```python
from build123d import *

# Parameters (mm, degrees)
ESQUISSE1_W                  = 220
ESQUISSE1_H                  = 200
BOSS_EXTRU_1_DEPTH           = 3
ESQUISSE2_R                  = 17.5
ENL_V_MAT_EXTRU_1_DEPTH      = 149.690954668
R_P_TITION_CIRCULAIRE1_COUNT = 6
R_P_TITION_CIRCULAIRE1_ANGLE = 120
EMPREINTE1_START             = 82
EMPREINTE1_OUTLINE_W         = 40
EMPREINTE1_OUTLINE_H         = 3
EMPREINTE1_DEPTH             = 3
EMPREINTE1_START_2           = 38.6
EMPREINTE1_2_OUTLINE_W       = 3
EMPREINTE1_2_OUTLINE_H       = 3
EMPREINTE1_2_DEPTH           = 33


# Read off the part's stored shape, not the designer's step: Empreinte1
with BuildPart() as part:
    # Esquisse1 → Boss.-Extru.1 (new body)
    with BuildSketch(Plane.XY):
        Rectangle(ESQUISSE1_W, ESQUISSE1_H)
    extrude(amount=BOSS_EXTRU_1_DEPTH)

    # Esquisse2 → Enlèv. mat.-Extru.1 (cut, through all)
    with BuildSketch(Plane.XY.offset(3)):
        with Locations((-86.602540378, -15)):
            Circle(ESQUISSE2_R)
    enl_v_mat_extru_1 = extrude(amount=-ENL_V_MAT_EXTRU_1_DEPTH, mode=Mode.SUBTRACT)

    # Répétition circulaire1: Enlèv. mat.-Extru.1 ×6 about axis
    r_p_tition_circulaire1_axis = Axis((0, 35, 0), (0, 0, 1))
    for i in range(1, R_P_TITION_CIRCULAIRE1_COUNT):
        add(enl_v_mat_extru_1.rotate(r_p_tition_circulaire1_axis, i * R_P_TITION_CIRCULAIRE1_ANGLE / (R_P_TITION_CIRCULAIRE1_COUNT - 1)), mode=Mode.SUBTRACT)

    # Empreinte1 outline → Empreinte1 (cut)
    with BuildSketch(Plane(origin=(0, 0, 0), x_dir=(1, 0, 0), z_dir=(0, 1, 0)).offset(EMPREINTE1_START)):
        with Locations((-53.7, -1.5)):
            Rectangle(EMPREINTE1_OUTLINE_W, EMPREINTE1_OUTLINE_H)
        with Locations((7.3, -1.5)):
            Rectangle(EMPREINTE1_OUTLINE_W, EMPREINTE1_OUTLINE_H)
    extrude(amount=EMPREINTE1_DEPTH, mode=Mode.SUBTRACT)

    # Empreinte1 2 outline → Empreinte1 2 (cut)
    with BuildSketch(Plane(origin=(0, 0, 0), x_dir=(1, 0, 0), z_dir=(0, 1, 0)).offset(EMPREINTE1_START_2)):
        with Locations((-92.2, -1.5)):
            Rectangle(EMPREINTE1_2_OUTLINE_W, EMPREINTE1_2_OUTLINE_H)
        with Locations((45.8, -1.5)):
            Rectangle(EMPREINTE1_2_OUTLINE_W, EMPREINTE1_2_OUTLINE_H)
    extrude(amount=EMPREINTE1_2_DEPTH, mode=Mode.SUBTRACT)


solid = part.part
```
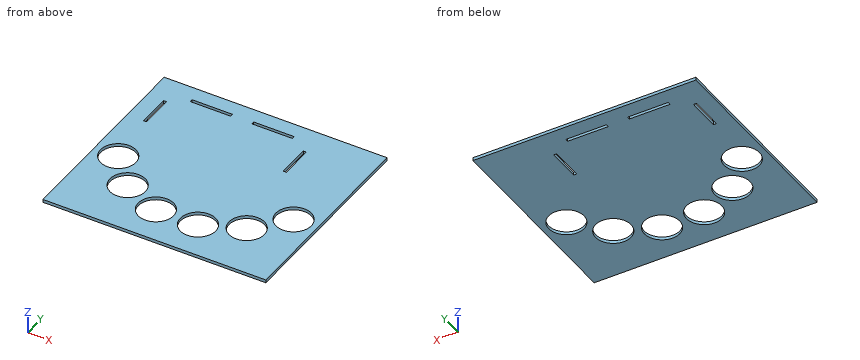
Geometry check sheet. Reference: the model listing, model coordinates, mm. Round coordinates to 2 decimals unless told otherwise and drop trailing zeros. Loops run counter-clockwise (first coordinate to the right, second up) from the corner with the lowest first, then second, coordinate; pieces in that order, holes last. Notation, with made-up numbers: M -19.5,-37.75 L 7.5,-37.75 A13 cw 7.5,-20.75 Z; hole C 71.5,52 d11. An arc over 180 degrees is marked long. Return JSON: item names as keys, results as strings. Group by question number.
(1) Section check B-B, the plane z = 1.25. Give the number of separate pieces and of enclosed holes in the cut face, and give its area (3 significant figures).
(2) Scan lines: line 1 along X through (y, z) = (47, 2.6); line 2 along Y through (x, z) = (10, 0.25); line 3 along Y through (x, z) = (-1.5, 2.8). Record each from-to range of solid material in increasing order. Write a range as [from, to].
(3) Section check A-A, the plane y = 56. Enter the section's corners in (x, z).
(4) Section check C-C, the plane x = 22. Enter the section's corners in (y, z), and give its area (3 significant figures).
(5) Section check D-D, the plane x = -26. Enter the section's corners in (y, z).
Data:
{
 "1": {"separate pieces": "1", "enclosed holes": "10", "area": "37,800 mm²"},
 "2": {"line 1": "[-110, -93.7], [-90.7, 44.3], [47.3, 110]", "line 2": "[-100, -76.59], [-49.04, 82], [85, 100]", "line 3": "[-100, 82], [85, 100]"},
 "3": {"outline": "M -110,0 L -93.7,0 L -93.7,3 L -110,3 Z; M -90.7,0 L 44.3,0 L 44.3,3 L -90.7,3 Z; M 47.3,0 L 110,0 L 110,3 L 47.3,3 Z"},
 "4": {"outline": "M -100,0 L -80.27,0 L -80.27,3 L -100,3 Z; M -45.36,0 L 82,0 L 82,3 L -45.36,3 Z; M 85,0 L 100,0 L 100,3 L 85,3 Z", "area": "486 mm²"},
 "5": {"outline": "M -100,0 L -79.52,0 L -79.52,3 L -100,3 Z; M -46.11,0 L 100,0 L 100,3 L -46.11,3 Z"}
}
